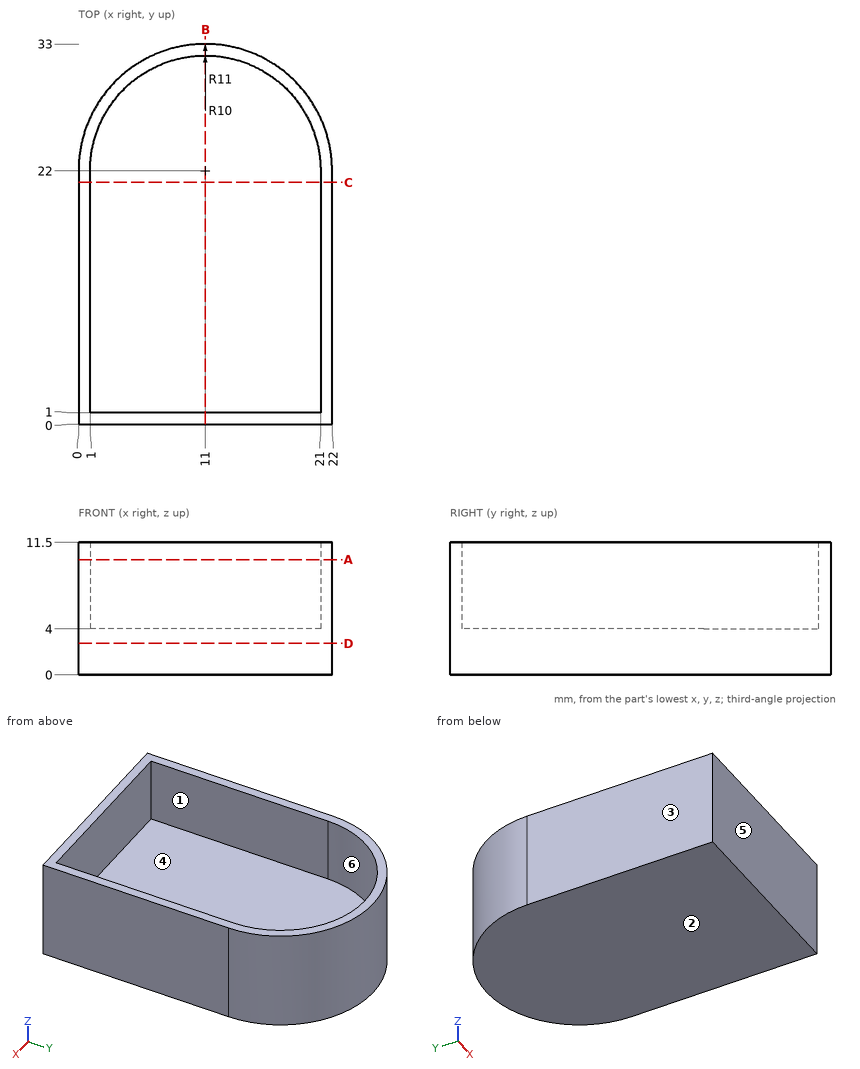
The figure shows three views and two pictorial views of one solid part (mm, origin at its lowest corner). Answer the questions. A direction names the side the tool comes from. Give positions to 0.01 mm unless a question says otherwise; leave off trailing zeros. Order: outer loops, then holes, each group sorted by start corner. A loop starts at its lowest first (then second) coordinate and runs counter-clockwise, first axis right, second up. Notation, with made-up numbers: (52.25, -21.5) -> (105.25, -21.5) arc R24 ccw to (105.25, 12.5) -> close; hole circle Ø5 at (20, 40.5). An arc over 180 degrees is marked (long way). Write each question's results on one line, items separated by ' | '.
Q1. The part is cut by section C-C, the plane y = 21. Give the vertices of the cut face in (x, z), and give its area (3 significant figures).
Checked values:
outline: (0, 0) -> (22, 0) -> (22, 11.5) -> (21, 11.5) -> (21, 4) -> (1, 4) -> (1, 11.5) -> (0, 11.5) -> close | area: 103 mm^2
Q2. Which of the six approach directions +Z, -Z, +X, -X, +Y, -Y give full straight-line access (tool end or side, diameter ignored) to the marked faces 1 and 2?
Checked values:
face 1: +Z | face 2: -Z, +X, -X, +Y, -Y
Q3. The part is cut by section A-A, the plane z = 10. Give the vertices of the cut face in (x, y).
Checked values:
outline: (0, 0) -> (22, 0) -> (22, 22) arc R11 ccw to (0, 22) -> close; hole (1, 1) -> (21, 1) -> (21, 22) arc R10 ccw to (1, 22) -> close
Q4. Each of these flat-tipped pins is pushed along its axis until it touches: P1, Ø5, axis at x = 15.5, z = 1.5, coming from the +Y side; P2, Ø1, axis at x = 16.5, y = 25, coming from the +Z side. Where does it stop, or does it pass through?
Checked values:
P1: stops at y = 32.82 | P2: stops at z = 4
Q5. The part is cut by section D-D, the plane z = 2.75. Give the vertices of the cut face in (x, y), and give its area (3 significant figures).
Checked values:
outline: (0, 0) -> (22, 0) -> (22, 22) arc R11 ccw to (0, 22) -> close | area: 674 mm^2
Q6. Determine the mould class of the marked faces 3, 4, 5 and 6 for opening direction X: pulls with the +X half, pulls with the -X half, needs draft (parallel to the pull), parting line crosses it, or undercut.
Checked values:
face 3: pulls with the -X half | face 4: undercut | face 5: needs draft | face 6: undercut
Q7. Straight lines are drawn through the part: probe 1 along Y at (x, z) = (11, 4.75); probe 2 along X at (y, z) = (19, 4.5); probe 3 along Z at (x, y) = (4.75, 17). For each, find the intervals that lie inside material, in ascending order. Write a range as from..to.
Checked values:
probe 1: y = 0..1, 32..33 | probe 2: x = 0..1, 21..22 | probe 3: z = 0..4
Q8. The part is cut by section B-B, the plane x = 11. Give the vertices of the cut face in (y, z), and give its area (3 significant figures).
Checked values:
outline: (0, 0) -> (33, 0) -> (33, 11.5) -> (32, 11.5) -> (32, 4) -> (1, 4) -> (1, 11.5) -> (0, 11.5) -> close | area: 147 mm^2
